Model file for the job. Use its own axes, mm. Give positions to 0.01 mm unless a question says otherwise; leave off trailing zeros. Order: outer loops, then holes, each group sorted by start corner. A loop starts at its lowest first (then second) coordinate and runs counter-clockwise, first axis right, second up. Notation, with made-up numbers: (-32, 28.25) - (-23, 28.25) arc R25 ccw to (-23, 57.25) - close; hole circle Ø11 at (-24.5, -23.75). An arc over 180 degrees is marked (long way). Return JSON: item names as keys, results as strings. Group by question number.
from build123d import *

# Parameters (mm, degrees)
F1_DEPTH = 19.05
F2_W     = 12.7
F2_H     = 406.4
F3_DEPTH = 9.525


# Not quite as in the source:
# - a feature names something its author has since deleted; it is built from what else it names


with BuildPart() as f1:
    # F0 (on Front) → F1 (new body)
    with BuildSketch(Plane.XZ):
        Polygon((-229.6549332498, 252.4134865394), (-356.6549332498, 252.4134865394), (-686.8549332498, 252.4134865394), (-686.8549332498, -153.9865134606), (-356.6549332498, -153.9865134606), (-26.4549332498, -153.9865134606), align=None)
    extrude(amount=F1_DEPTH)

    # F2 (on face) → F3 (cut)
    with BuildSketch(Plane(origin=(0, 0, 0), x_dir=(-1, 0, 0), z_dir=(0, 1, 0))):
        with Locations((388.4049332498, 49.2134865394)):
            Rectangle(F2_W, F2_H)
    extrude(amount=-F3_DEPTH, mode=Mode.SUBTRACT)


solid = f1.part
(1) Pull direction X, two halves, no side cores. Call faces 1 (the face through (-455, -9, 252.413)), 2 (the face through (-686.855, -9, 52)), 3 (the face through (-388, -9.525, 52)): released by +X, released by -X, zero draft, split by the parting line, or undercut.
(2) Drop flat-ended pins along their axis: pin 1 Ø3 at (y, z) = (-7, 96) entering from +X; pin 2 Ø10 at (y, z) = (-7.5, 42) entering from +X; pin 3 Ø1.5 at (y, z) = (-11.5, -38.5) entering from +X. Give the stop position or say it passes through.
(3) Slice it at D-D (z = -34). Give the cut face in (x, y) (3 decimals).
(4) Slice it at A-A (y = -3.5). Give the cut face in (x, z).
(5) Slice it at C-C (x = -99.5). Give the cut face in (y, z), and give its area (3 significant figures).
(6) Slice it at B-B (z = 188). Give the cut face in (x, y) (3 decimals), and give its area (3 significant figures).
(7) Drill centre lines: L1, parallel to X at y = -6.5, z = -19.5; L2, parallel to X at y = -6.5, z = 97.5; L3, parallel to Z at x = -118.5, y = -9. Where is each one in solid material? Low to high.
Result set:
{
 "1": {"face 1": "zero draft", "face 2": "released by -X", "face 3": "undercut"},
 "2": {"pin 1": "stops at x = -150.7", "pin 2": "stops at x = -121.95", "pin 3": "stops at x = -83.82"},
 "3": {"outline": "(-686.855, -19.05) - (-86.448, -19.05) - (-86.448, 0) - (-382.055, 0) - (-382.055, -9.525) - (-394.755, -9.525) - (-394.755, 0) - (-686.855, 0) - close"},
 "4": {"outline": "(-686.85, -153.99) - (-394.75, -153.99) - (-394.75, 252.41) - (-686.85, 252.41) - close; (-382.05, -153.99) - (-26.45, -153.99) - (-229.65, 252.41) - (-382.05, 252.41) - close"},
 "5": {"outline": "(-19.05, -153.99) - (0, -153.99) - (0, -7.9) - (-19.05, -7.9) - close", "area": "2,780 mm²"},
 "6": {"outline": "(-686.855, -19.05) - (-197.448, -19.05) - (-197.448, 0) - (-382.055, 0) - (-382.055, -9.525) - (-394.755, -9.525) - (-394.755, 0) - (-686.855, 0) - close", "area": "9,200 mm²"},
 "7": {"L1": "x = -686.85 to -394.75, -382.05 to -93.7", "L2": "x = -686.85 to -394.75, -382.05 to -152.2", "L3": "z = -153.99 to 30.1"}
}
